Can you work these out from the model? Positions are in its coordinate system, mm. Give positions to 0.01 mm unless a question says otherwise; leave off trailing zeros. Loops run counter-clockwise (first coordinate to the right, second up) from the corner with the lowest first, then second, coordinate; pieces in that order, holes last. Notation, with made-up numbers: M -5,-26 L 25,-26 A23 ccw 25,9 Z; hole C 7,-16.75 d9. An arc over 180 degrees is marked long. Put each result on its own line as item: value. Start each with the question number.
1) Imagine slicing it at B-B (y = -218). Write out the boundary of the cut face in (x, z).
2) Please list where these lines run through material, in increasing order: line 1 along X through (y, z) = (-149, 10.75); line 2 along Z through (x, y) = (22, -159); line 3 along X through (y, z) = (-277, 13.25). Write a range as from..to.
3) Imagine slicing it at A-A (x = 23.75). Write out the boundary of the cut face in (y, z).
4) For P1, Ø5, axis at x = 27, z = 10, coming from the +Y side, with a flat end and sliding along its axis, tell me the tip position at first contact or that it passes through.
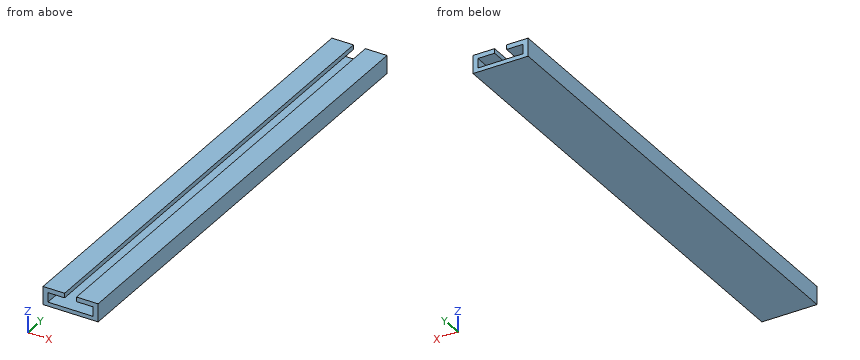
Autodesk Inventor part; units mm, degrees
ref_plane "YZ Plane" through (0, 0, 0) normal (1, 0, 0) x (0, 1, 0)
ref_plane "XZ Plane" through (0, 0, 0) normal (0, 1, 0) x (-1, 0, 0)
ref_plane "XY Plane" through (0, 0, 0) normal (0, 0, 1) x (1, 0, 0)
sketch "Sketch1" plane through (0, 0, 0) normal (0, 0, 1) x (1, 0, 0)
  line L0 (-15.9487, -92.7565) -> (47.5513, -92.7565)
  line L1 (47.5513, -92.7565) -> (47.5513, -346.7565)
  line L2 (47.5513, -346.7565) -> (-15.9487, -346.7565)
  line L3 (-15.9487, -346.7565) -> (-15.9487, -92.7565)
  point P0 (0, 0)
  dimension "d0" = 63.5
  dimension "d2" = 254
extrude "Extrusion1" add sketch "Sketch1" along normal blind 19.05
sketch "Sketch2" plane through (-15.9487, -92.7565, 0) normal (0, 1, 0) x (1, 0, 0)
  point P0 (15.9487, 0)
sketch "Sketch3" plane through (-15.9487, -92.7565, 0) normal (0, 1, 0) x (1, 0, 0)
  line L0 (63.5, -19.05) -> (0, -19.05)
  line L1 (34.925, -19.05) -> (28.575, -19.05)
  line L2 (28.575, -19.05) -> (28.575, -12.0642)
  line L3 (34.925, -12.0642) -> (34.925, -19.05)
  line L4 (31.75, -19.05) -> (31.75, 0) construction
  line L5 (63.5, 0) -> (63.5, -19.05)
  line L6 (28.575, -12.0642) -> (19.685, -12.0642)
  line L7 (19.685, -12.0642) -> (19.685, -6.9842)
  line L8 (19.685, -6.9842) -> (28.575, -6.9842)
  line L9 (34.925, -12.0642) -> (43.815, -12.0642)
  line L10 (43.815, -12.0642) -> (43.815, -6.9842)
  line L11 (43.815, -6.9842) -> (34.925, -6.9842)
  line L12 (34.925, -6.9842) -> (28.575, -6.9842)
  point P0 (15.9487, 0)
  dimension "d6" = 31.75
  dimension "d7" = 8.89
  dimension "d8" = 5.08
  dimension "d9" = 8.89
extrude "Extrusion2" cut sketch "Sketch3" against normal blind 254
sketch "Sketch4" plane through (-15.9487, -92.7565, 0) normal (0, 1, 0) x (1, 0, 0)
  line L0 (63.5, 0) -> (63.5, -19.05)
  line L1 (63.5, 0) -> (46.4201, 0)
  line L2 (46.4201, 0) -> (46.4201, -19.05)
  line L3 (46.4201, -19.05) -> (63.5, -19.05)
  line L4 (63.5, -19.05) -> (63.5, 0)
  line L5 (63.5, 0) -> (0, 0)
  line L6 (31.75, 0) -> (31.75, -19.05) construction
  line L7 (0, 0) -> (0, -19.05)
  line L8 (0, 0) -> (17.0799, 0)
  line L9 (17.0799, 0) -> (17.0799, -19.05)
  line L10 (0, -19.05) -> (17.0799, -19.05)
  point P0 (15.9487, 0)
extrude "Extrusion3" cut sketch "Sketch4" against normal blind 254
sketch "Sketch5" plane through (3.7363, -92.7565, 6.9842) normal (0, 1, 0) x (1, 0, 0)
  line L0 (-2.6051, 6.9842) -> (-2.6051, -12.0658)
  line L1 (26.7351, 6.9842) -> (26.7351, -12.0658)
  line L2 (-2.6051, 6.9842) -> (26.7351, 6.9842)
  line L3 (26.7351, 6.9842) -> (26.7351, 2.1306)
  line L4 (26.7351, 2.1306) -> (-2.6051, 2.1306)
  line L5 (-2.6051, 2.1306) -> (-2.6051, 6.9842)
  point P0 (-3.7363, 6.9842)
extrude "Extrusion4" cut sketch "Sketch5" against normal blind 254
sketch "Sketch6" plane through (3.7363, -92.7565, 6.9842) normal (0, 1, 0) x (1, 0, 0)
  line L0 (-2.6051, -12.0658) -> (-2.6051, 2.1306)
  line L1 (26.7351, 2.1306) -> (26.7351, -12.0658)
  line L2 (-2.6051, -12.0658) -> (26.7351, -12.0658)
  line L3 (26.7351, -12.0658) -> (26.7351, -7.5248)
  line L4 (26.7351, -7.5248) -> (-2.6051, -7.5248)
  line L5 (-2.6051, -7.5248) -> (-2.6051, -12.0658)
  point P0 (-3.7363, 6.9842)
extrude "Extrusion5" cut sketch "Sketch6" against normal blind 254
properties part number "crossbowtrack"
Recorded:
1. outline: M 1.13,4.85 L 30.47,4.85 L 30.47,14.51 L 18.98,14.51 L 18.98,12.06 L 27.87,12.06 L 27.87,6.98 L 3.74,6.98 L 3.74,12.06 L 12.63,12.06 L 12.63,14.51 L 1.13,14.51 Z
2. line 1: 1.13..3.74, 27.87..30.47
2. line 2: 4.85..6.98, 12.06..14.51
2. line 3: 1.13..12.63, 18.98..30.47
3. outline: M -346.76,4.85 L -92.76,4.85 L -92.76,6.98 L -346.76,6.98 Z; M -346.76,12.06 L -92.76,12.06 L -92.76,14.51 L -346.76,14.51 Z
4. P1: y = -92.76
